Drawing for the job (mm, zero at the part's lowest x, y, z). Give positions to 0.01 mm unless a question says otherwise; leave off trailing zeros. Order: outer loops, then holes, each group sorted by start corner. A loop starts at its lowest first (then second) coordinate and runs counter-clockwise, first axis right, second up. Notation, with made-up numbers: M 25,-27 L 73,-27 A22 ccw 73,2 Z; hole C -23.5,-11.5 d6. An arc over 180 degrees is marked long. One line per item, written item: value.
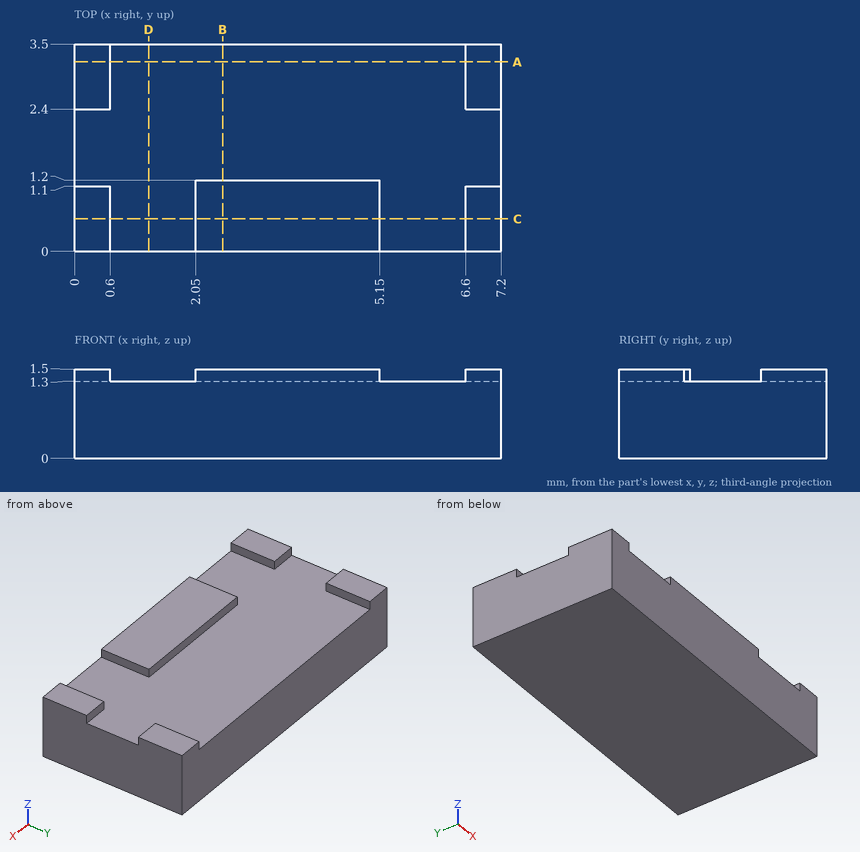
1) Saw through at A-A, the plane y = 3.2. Write the cut outline in (x, z).
Check values:
outline: M 0,0 L 7.2,0 L 7.2,1.5 L 6.6,1.5 L 6.6,1.3 L 0.6,1.3 L 0.6,1.5 L 0,1.5 Z
2) Drill centre lines: probe 1 along X at (y, z) = (3, 1.4); probe 2 along X at (y, z) = (0.9, 1.4); probe 3 along Z at (x, y) = (4, 3.15). Where is each one in solid material? Low to high. Write a range as from..to.
Check values:
probe 1: 0..0.6, 6.6..7.2
probe 2: 0..0.6, 2.05..5.15, 6.6..7.2
probe 3: 0..1.3
3) Saw through at D-D, the plane x = 1.25. Write the cut outline in (y, z).
Check values:
outline: M 0,0 L 3.5,0 L 3.5,1.3 L 0,1.3 Z
4) Saw through at B-B, the plane x = 2.5. Write the cut outline in (y, z).
Check values:
outline: M 0,0 L 3.5,0 L 3.5,1.3 L 1.2,1.3 L 1.2,1.5 L 0,1.5 Z
5) Saw through at C-C, the plane y = 0.55. Write the cut outline in (x, z), then the cut area to 3 significant figures.
Check values:
outline: M 0,0 L 7.2,0 L 7.2,1.5 L 6.6,1.5 L 6.6,1.3 L 5.15,1.3 L 5.15,1.5 L 2.05,1.5 L 2.05,1.3 L 0.6,1.3 L 0.6,1.5 L 0,1.5 Z
area: 10.2 mm^2
6) Pin check, flat tip, straight feed: pin 1 (1.8 mm diameter, centred on x = 5, y = 2.5, fed in from +Z). Stop position of the tip, or through.
Check values:
pin 1: z = 1.3
